Input: dimensioned drawing with shaded views. Units: mm. Origin: part minimum x, y, z. Coordinates: 2 decimals unless noted, no trailing zeros. Order: outer loops, then holes, each group sorted by start corner. A loop starts at its lowest first (then second) coordinate and runs counter-clockwise, first axis right, second up.
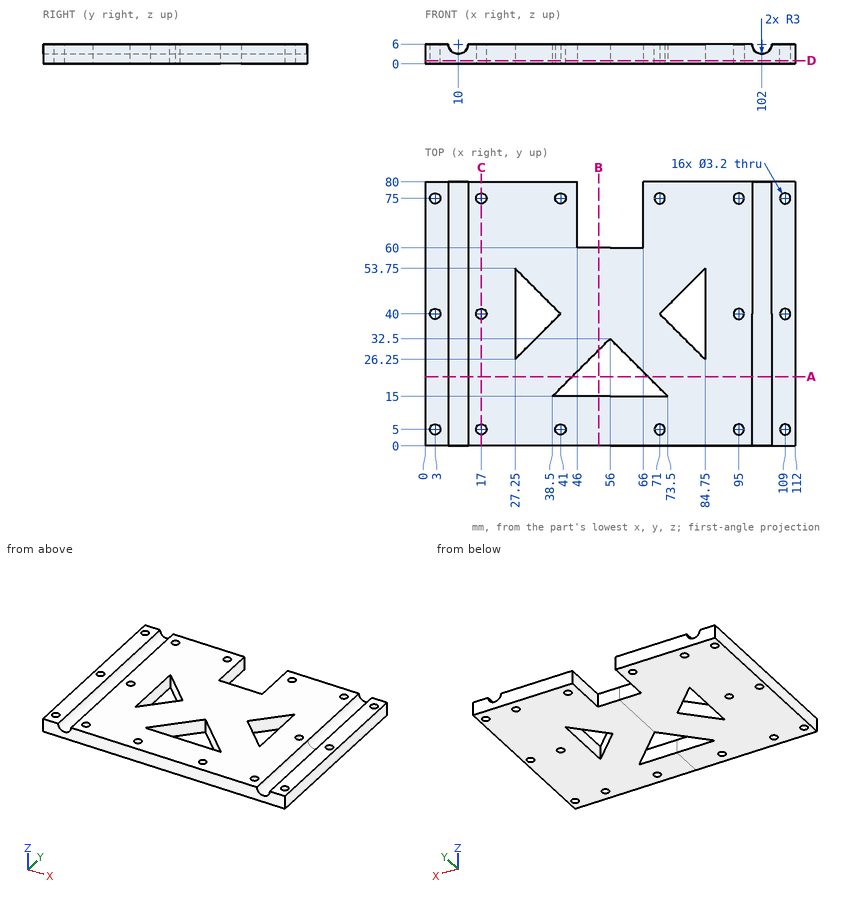
1. Contact query for flat-ended pins moving along their axis: P1, Ø2.5, axis at x = 109, y = 5, coming from the +Z side; P2, Ø1.5, axis at x = 61.5, z = 2, coming from the +Y side. Output: stop coordinate, or through.
2. Material intervals for line 1 along Y through (x, z) = (3, 4); line 2 along X through (y, z) = (46, 5.2); line 3 along X through (y, z) = (71, 5.25), sorted ascending.
3. Section query C-C, the plane x = 17. Output: boundary loops of the cut face in (y, z).
4. Section query B-B, the plane x = 52.5. Output: boundary loops of the cut face in (y, z).
5. Section query A-A, the plane y = 21. Output: boundary loops of the cut face in (x, z), plus the area to 3 significant figures.
6. Section query D-D, the plane z = 1. Count the separate pieces of the cut face and the enclosed holes in it, plus the area to 3 significant figures.
Answer key:
1. P1: passes through
1. P2: stops at y = 60
2. line 1: y = 0 to 3.4, 6.6 to 38.4, 41.6 to 73.4, 76.6 to 80
2. line 2: x = 0 to 7.11, 12.89 to 27.25, 35 to 77, 84.75 to 99.11, 104.89 to 112
2. line 3: x = 0 to 7.1, 12.9 to 46, 66 to 99.1, 104.9 to 112
3. outline: (0, 0) - (3.4, 0) - (3.4, 6) - (0, 6) - close; (6.6, 0) - (38.4, 0) - (38.4, 6) - (6.6, 6) - close; (41.6, 0) - (73.4, 0) - (73.4, 6) - (41.6, 6) - close; (76.6, 0) - (80, 0) - (80, 6) - (76.6, 6) - close
4. outline: (0, 0) - (15, 0) - (15, 6) - (0, 6) - close; (29, 0) - (60, 0) - (60, 6) - (29, 6) - close
5. outline: (0, 0) - (44.5, 0) - (44.5, 6) - (13, 6) arc R3 cw to (7, 6) - (0, 6) - close; (67.5, 0) - (112, 0) - (112, 6) - (105, 6) arc R3 cw to (99, 6) - (67.5, 6) - close
5. area: 506 mm2
6. separate pieces: 1
6. enclosed holes: 19
6. area: 7,750 mm2
